Input: part model. Units: mm. Frame: model coordinates. Face numbers are marked on the shaded views. A direction names the side the tool comes from. Give positions to 0.01 mm unless a question says otherwise; leave off trailing zeros. Loops run counter-clockwise (first coordinate to the right, second up) from the corner with the lowest first, then second, coordinate; pieces in that order, holes last. Notation, with made-up numbers: M 81.25,-9.5 L 128.25,-9.5 A24 cw 128.25,22.5 Z; hole C 26,10.5 d6. An arc over 180 degrees is marked long. Return JSON: item names as keys, results as strings. Group by question number.
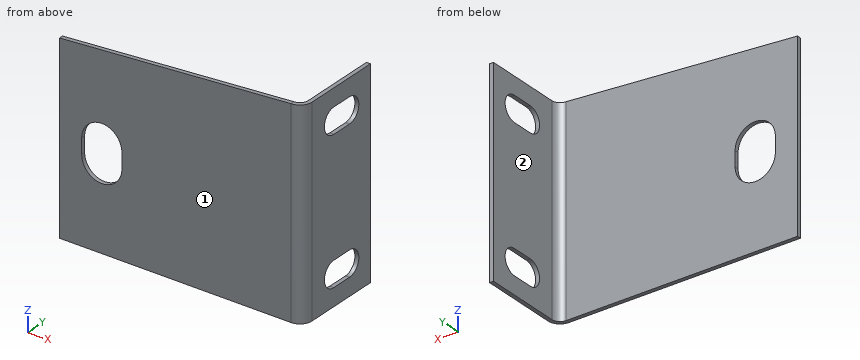
```python
from build123d import *

# Parameters (mm, degrees)
EXTRUDE_THIN1_DEPTH = 25.4
CUT_EXTRUDE1_DEPTH  = 42.405263868
CUT_EXTRUDE2_DEPTH  = 42.33848541


with BuildPart() as part:
    # Sketch3 → Extrude-Thin1 (new body)
    with BuildSketch(Plane.XY):
        with BuildLine():
            Line((0, -0.25), (29.21, -0.25))
            ThreePointArc((29.21, -0.25), (30.284802307, 0.195197693), (30.73, 1.27))
            Line((30.73, 1.27), (30.73, 11.176))
            Line((30.73, 11.176), (30.23, 11.176))
            Line((30.23, 11.176), (30.23, 1.27))
            ThreePointArc((30.23, 1.27), (29.931248917, 0.548751083), (29.21, 0.25))
            Line((29.21, 0.25), (0, 0.25))
            Line((0, 0.25), (0, -0.25))
        make_face()
    extrude(amount=EXTRUDE_THIN1_DEPTH)

    # Sketch4 → Cut-Extrude1 (cut, through all)
    with BuildSketch(Plane(origin=(30.73, 0, 0), x_dir=(0, 0, -1), z_dir=(1, 0, 0))):
        with BuildLine():
            Line((-5.3975, 4.953), (-5.3975, 7.62))
            ThreePointArc((-5.3975, 7.62), (-3.81, 9.2075), (-2.2225, 7.62))
            Line((-2.2225, 7.62), (-2.2225, 4.953))
            ThreePointArc((-2.2225, 4.953), (-3.81, 3.3655), (-5.3975, 4.953))
        make_face()
        with BuildLine():
            Line((-20.0025, 4.953), (-20.0025, 7.62))
            ThreePointArc((-20.0025, 7.62), (-21.59, 9.2075), (-23.1775, 7.62))
            Line((-23.1775, 7.62), (-23.1775, 4.953))
            ThreePointArc((-23.1775, 4.953), (-21.59, 3.3655), (-20.0025, 4.953))
        make_face()
    extrude(amount=-CUT_EXTRUDE1_DEPTH, mode=Mode.SUBTRACT)

    # Sketch5 → Cut-Extrude2 (cut, through all)
    with BuildSketch(Plane(origin=(0, 0.25, 0), x_dir=(1, 0, 0), z_dir=(0, 1, 0))):
        with BuildLine():
            Line((2.794, -12.573), (2.794, -10.668))
            ThreePointArc((2.794, -10.668), (5.334, -8.128), (7.874, -10.668))
            Line((7.874, -10.668), (7.874, -12.573))
            ThreePointArc((7.874, -12.573), (5.334, -15.113), (2.794, -12.573))
        make_face()
        Polygon((29.21, -25.4), (0, -25.4), (0, -23.241), align=None)
    extrude(amount=-CUT_EXTRUDE2_DEPTH, mode=Mode.SUBTRACT)


solid = part.part
```
Item 1: Material intervals for line 1 (Y direction, x = 23.5, z = 20.5); line 2 (X direction, y = 3, z = 11.25), sorted ascending. Write a range as from..to.
Item 2: Reachability of the marked faces 1 and 2 from +Z, -Z, +X, -X, +Y, -Y: full face, straight path, thin tool, end or side. Return the list, or none.
Item 3: Section C-C, the plane y = 4.25. Return loops of the section in (x, z), then the cut area to 3 significant figures.
Item 4: Section B-B, the plane x = 4. Return loops of the section in (y, z).
Item 5: Section D-D, the plane z = 7.25. Return loops of the section in (x, y), then the cut area to 3 significant figures.
Item 6: First-contact query: pin 1 Ø8 at (x, z) = (10.5, 15.5) entering from +Y; pin 2 Ø6 at (y, z) = (8.5, 19.5) entering from -X; pin 3 Ø2 at (x, y) = (27.5, 1.5) entering from -Z. Flat tips, straight axial feed; report the tip coordinate or a pass-through.
Item 7: Section A-A, the plane z = 21.59. Return loops of the section in (x, y), then the cut area to 3 significant figures.
Answer below:
{
 "1": {"line 1": "-0.25..0.25", "line 2": "30.23..30.73"},
 "2": {"face 1": "+Z, -Z, +X, -X, -Y", "face 2": "+Z, -Z, -X, +Y"},
 "3": {"outline": "M 30.23,0 L 30.73,0 L 30.73,2.39 L 30.23,2.39 Z; M 30.23,5.23 L 30.73,5.23 L 30.73,20.17 L 30.23,20.17 Z; M 30.23,23.01 L 30.73,23.01 L 30.73,25.4 L 30.23,25.4 Z", "area": "9.85 mm^2"},
 "4": {"outline": "M -0.25,0 L 0.25,0 L 0.25,8.51 L -0.25,8.51 Z; M -0.25,14.73 L 0.25,14.73 L 0.25,23.54 L -0.25,23.54 Z"},
 "5": {"outline": "M 0,-0.25 L 29.21,-0.25 A1.52 ccw 30.73,1.27 L 30.73,11.18 L 30.23,11.18 L 30.23,1.27 A1.02 cw 29.21,0.25 L 0,0.25 Z", "area": "20.6 mm^2"},
 "6": {"pin 1": "y = 0.25", "pin 2": "x = 30.23", "pin 3": "through"},
 "7": {"outline": "M 0,-0.25 L 29.21,-0.25 A1.52 ccw 30.73,1.27 L 30.73,3.37 L 30.23,3.37 L 30.23,1.27 A1.02 cw 29.21,0.25 L 0,0.25 Z; M 30.23,9.21 L 30.73,9.21 L 30.73,11.18 L 30.23,11.18 Z", "area": "17.6 mm^2"}
}
